Autodesk Inventor part; units mm, degrees
ref_plane "XZ Plane" through (0, 0, 0) normal (0, 1, 0) x (-1, 0, 0)
ref_plane "XY Plane" through (0, 0, 0) normal (0, 0, 1) x (1, 0, 0)
sketch "Skizze1" plane through (0, 0, 0) normal (0, 1, 0) x (-1, 0, 0)
  circle A0 centre (0, 0) radius 28.5
  dimension "d0" = 57
extrude "Extrusion1" add sketch "Skizze1" along normal blind 9
sketch "Skizze2" plane through (0, 0, 0) normal (0, -1, 0) x (1, 0, 0)
  circle A0 centre (0, 0) radius 10
  dimension "d3" = 20
extrude "Extrusion2" add sketch "Skizze2" along normal blind 9
sketch "Skizze3" plane through (0, 9, 0) normal (0, 1, 0) x (1, 0, 0)
  circle A0 centre (0, -22) radius 4
  point P0 (0, 0)
  dimension "d6" = 8
extrude "Extrusion3" add sketch "Skizze3" along normal blind 13
sketch "Skizze4" plane through (0, 0, 0) normal (1, 0, 0) x (0, 1, 0)
  circle A0 centre (-4.5, 0) radius 2
  point P0 (0, 0)
  dimension "d9" = 4
extrude "Extrusion4" cut sketch "Skizze4" along normal mid plane 25
sketch "Skizze5" plane through (0, -9, 0) normal (0, -1, 0) x (1, 0, 0)
  circle A0 centre (0, 0) radius 5.5
  dimension "d12" = 11
extrude "Extrusion5" cut sketch "Skizze5" against normal up to surface (18 mm away)
fillet "Rundung1" radius 0.5 5 edges at (28.5, 9, 0) (28.5, 0, 0) (-10, 0, 0) (-10, -9, 0) (-4, 22, 22)
properties part number "sf_Crank_Disc_1"
For this review, take the finished solid that the model builds, in its own axes (mm). A direction names the side the tool comes from. Round coordinates to 2 decimals unless told otherwise and drop trailing zeros. Order: outer loops, then holes, each group sorted by start corner. A loop starts at its lowest first (then second) coordinate and runs counter-clockwise, first axis right, second up.
Q1. We need section D-D, the plane y = 15. Give the boundary of the cut face in (x, z), plus the area to 3 significant figures.
Findings below:
outline: circle Ø8 at (0, 22)
area: 50.3 mm2
Q2. We need section B-B, the plane x = 0. Give the boundary of the cut face in (y, z).
Findings below:
outline: (-9, -9.5) arc R0.5 ccw to (-8.5, -10) - (-0.5, -10) arc R0.5 cw to (0, -10.5) - (0, -28) arc R0.5 ccw to (0.5, -28.5) - (8.5, -28.5) arc R0.5 ccw to (9, -28) - (9, -5.5) - (-9, -5.5) - close; (-9, 5.5) - (9, 5.5) - (9, 18) - (21.5, 18) arc R0.5 ccw to (22, 18.5) - (22, 25.5) arc R0.5 ccw to (21.5, 26) - (9, 26) - (9, 28) arc R0.5 ccw to (8.5, 28.5) - (0.5, 28.5) arc R0.5 ccw to (0, 28) - (0, 10.5) arc R0.5 cw to (-0.5, 10) - (-8.5, 10) arc R0.5 ccw to (-9, 9.5) - close
Q3. Machinability: for faces 4 (the cylindrical face through (-7.528, -4.76, 1.983)), 5 (the cylindrical face through (-0.521, 15.162, 25.966)), 6 (the cylindrical face through (9.237, -4.444, 3.83)), which of the approach directions +Z, -Z, +X, -X, +Y, -Y give a long, thin tool a straight path to every point of the face, cutting with its end or side? Answer none if there is none.
Findings below:
face 4: +X, -X
face 5: +Y
face 6: -Y
Q4. We need section A-A, the plane z = 0. Give the boundary of the cut face in (x, y), plus the area to 3 significant figures.
Findings below:
outline: (-28.5, 0.5) arc R0.5 ccw to (-28, 0) - (-10.5, 0) arc R0.5 cw to (-10, -0.5) - (-10, -2.5) - (-5.5, -2.5) - (-5.5, 9) - (-28, 9) arc R0.5 ccw to (-28.5, 8.5) - close; (-10, -8.5) arc R0.5 ccw to (-9.5, -9) - (-5.5, -9) - (-5.5, -6.5) - (-10, -6.5) - close; (5.5, -9) - (9.5, -9) arc R0.5 ccw to (10, -8.5) - (10, -6.5) - (5.5, -6.5) - close; (5.5, -2.5) - (10, -2.5) - (10, -0.5) arc R0.5 cw to (10.5, 0) - (28, 0) arc R0.5 ccw to (28.5, 0.5) - (28.5, 8.5) arc R0.5 ccw to (28, 9) - (5.5, 9) - close
area: 459 mm2
Q5. Insertion check: P1, Ø5, axis at y = 0, z = 9.5, coming from the +X side; P2, Ø1.5, axis at x = 10.5, z = -19, coming from the +Y side; P3, Ø6.5, axis at y = -4.5, z = 0, coming from the -X side. Each pin has a flat end and moves straight along its axis. Give the tip position at first contact, or say it passes through.
Findings below:
P1: stops at x = 27.61
P2: stops at y = 9
P3: stops at x = -10
Q6. Mouldability with a two-part tool opening along X and no side actions: class faces 1 (the cylindrical face through (-26.327, 4.444, 10.916)), 2 (the flat face through (4, -9, -4)), 3 (the cylindrical face through (5.08, -0.13, -2.11)) as pulls with the +X half, pulls with the -X half, needs draft (parallel to the pull), parting line crosses it, or undercut.
Findings below:
face 1: parting line crosses it
face 2: needs draft
face 3: undercut
Q7. Wall thickness on line 1 (Z direction, x = 0, y = 5.25); line 2 (Z direction, x = 0, y = -2); line 3 (Y direction, x = -18.5, z = -18): over which ranges is each line inside the solid? List them lowest first.
Findings below:
line 1: z = -28.5 to -5.5, 5.5 to 28.5
line 2: z = -10 to -5.5, 5.5 to 10
line 3: y = 0 to 9
Q8. We need section C-C, the plane y = -4.5. Give the boundary of the cut face in (x, z).
Findings below:
outline: (-9.8, -2) arc R10 ccw to (9.8, -2) - (5.12, -2) arc R5.5 cw to (-5.12, -2) - close; (-9.8, 2) - (-5.12, 2) arc R5.5 cw to (5.12, 2) - (9.8, 2) arc R10 ccw to start
